from build123d import *

# Parameters (mm, degrees)
F1_DEPTH        = 34.5
F2_R            = 12.5
F3_DEPTH        = 4.1
F4_R            = 13
F5_DEPTH        = 4.1
F6_W            = 20.7
F6_H            = 29.8
F6_H_2          = 0.9
F7_DEPTH        = 31.9
F10_D           = 1.5
F10_DEPTH       = 5
F10_TIP         = 0.4506454643
F10_ON_F9_D     = 1.5
F10_ON_F9_DEPTH = 5
F10_ON_F9_TIP   = 0.4506454643
F12_DEPTH       = 25


with BuildPart() as f1:
    # F0 (on Front) → F1 (new body)
    with BuildSketch(Plane.XZ):
        Polygon((0, 36), (0, 0), (36, 0), (36, 5), (5, 36), align=None)
    extrude(amount=F1_DEPTH)

    # F2 (on face) → F3 (cut)
    with BuildSketch(Plane(origin=(0, 0, 0), x_dir=(0, -1, 0), z_dir=(-1, 0, 0))):
        with Locations((17.25, 18)):
            Circle(F2_R)
    extrude(amount=-F3_DEPTH, mode=Mode.SUBTRACT)

    # F4 (on face) → F5 (cut)
    with BuildSketch(Plane(origin=(0, 0, 0), x_dir=(1, 0, 0), z_dir=(0, 0, -1))):
        with Locations((18, 17.25)):
            Circle(F4_R)
    extrude(amount=-F5_DEPTH, mode=Mode.SUBTRACT)

    # F6 (on face) → F7 (cut)
    with BuildSketch(Plane.YZ.offset(36)):
        with Locations((-17.25, 19.9)):
            Rectangle(F6_W, F6_H)
        with Locations((-17.25, 4.55)):
            Rectangle(F6_W, F6_H_2)
    extrude(amount=-F7_DEPTH, mode=Mode.SUBTRACT)

    # F10
    with Locations(Plane.XY.offset(36)):
        with Locations((2.75, -31.75), (2.75, -2.75)):
            Hole(F10_D / 2, depth=F10_DEPTH)
            with Locations((0, 0, -(F10_DEPTH + F10_TIP / 2))):  # 118° drill point
                Cone(0, F10_D / 2, F10_TIP, mode=Mode.SUBTRACT)

    # F10 on F9
    with Locations(Plane.YZ.offset(36)):
        with Locations((-31.75, 2.75), (-2.75, 2.75)):
            Hole(F10_ON_F9_D / 2, depth=F10_ON_F9_DEPTH)
            with Locations((0, 0, -(F10_ON_F9_DEPTH + F10_ON_F9_TIP / 2))):  # 118° drill point
                Cone(0, F10_ON_F9_D / 2, F10_ON_F9_TIP, mode=Mode.SUBTRACT)

    # F11 (on face) → F12 (cut)
    with BuildSketch(Plane(origin=(0, 0, 0), x_dir=(0, -1, 0), z_dir=(-1, 0, 0))):
        with BuildLine():
            ThreePointArc((18, 5.5225202865), (17.5002003207, 5.5025042589), (17, 5.5025002501))
            Line((17, 5.5025002501), (17, 0))
            Line((17, 0), (18, 0))
            Line((18, 0), (18, 5.5225202865))
        make_face()
    extrude(amount=-F12_DEPTH, mode=Mode.SUBTRACT)


solid = f1.part
Design review of the part built by this model. Coordinates are the model's own, in mm. A direction names the side the tool comes from. Coordinates: 2 decimals unless noted, no trailing zeros. Order: outer loops, then holes, each group sorted by start corner. A loop starts at its lowest first (then second) coordinate and runs counter-clockwise, first axis right, second up. Notation, with made-up numbers: (46.25, 66.25) -> (52.25, 66.25) arc R31 ccw to (52.25, 93.25) -> close; hole circle Ø9 at (37, 2). An arc over 180 degrees is marked (long way). Use one line per item in the form item = value. Start each with the question number.
(1) Add section A-A on x = 18. State the section outline as (y, z) points.
(2) Add section C-C on y = -21.5. State the section outline as (x, z) points.
(3) Insertion check: pin 1 (8 mm diameter, centred on x = 32.5, y = -19.5, fed in from +Z); pin 2 (0.6 mm diameter, centred on y = -6, z = 15.5, fed in from -X); pin 3 (6 mm diameter, centred on x = 20, y = -7, fed in from +Z); pin 4 (3 mm diameter, centred on x = 31.5, z = 12, fed in from +Y). Each pin has a flat end and moves straight along its axis. Give the tip position at first contact, or say it passes through.
(4) For faces 5 (the flat face through (17, -27.6, 16)), 6 (the flat face through (2, -18, 3)), 7 (the flat face through (18, -29, 4.1)), 8 (the flat face through (4.1, -6, 18)), list the 3-axis set-ups (+Z, -Z, +X, -X, +Y, -Y) from which the entire face can be reached by the end or side of a thin tool; tool diameter is ignored.
(5) The part is to be moulded in two halves that separate along Z. For faces 1 (the flat face through (32, -17, 4.1)), 2 (the flat face through (18, -6, 4.1)), 3 (the cylindrical face through (33.465, -32.465, 2.975)), 4 (the flat face through (0, -13, 30)), say which applies: +Z half, -Z half, draft (parallel to the pull), parting line (faces both ways), or undercut.
(6) Add section B-B on z = 18. State the section outline as (x, y) points.
(7) Add section D-D on y = -14.5. State the section outline as (x, z) points, plus the area to 3 significant figures.
(8) For probe 1 along Y at (x, z) = (2.75, 34.05); probe 2 along Y at (x, z) = (16, 12); probe 3 along X at (y, z) = (-0.5, 16), list the stretches that pass through material, from the lowest coordinate up.
Answer block:
q1.outline = (-34.5, 0) -> (-30.25, 0) -> (-30.25, 4.1) -> (-27.6, 4.1) -> (-27.6, 23) -> (-34.5, 23) -> close; (-6.9, 4.1) -> (-4.25, 4.1) -> (-4.25, 0) -> (0, 0) -> (0, 23) -> (-6.9, 23) -> close
q2.outline = (0, 0) -> (5.71, 0) -> (5.71, 4.1) -> (4.1, 4.1) -> (4.1, 6.24) -> (0, 6.24) -> close; (0, 29.76) -> (4.1, 29.76) -> (4.1, 34.8) -> (6.2, 34.8) -> (5, 36) -> (0, 36) -> close; (30.29, 0) -> (36, 0) -> (36, 4.1) -> (30.29, 4.1) -> close
q3.pin_1 = 4.1
q3.pin_2 = 4.1
q3.pin_3 = 24
q3.pin_4 = through
q4.face_5 = +X
q4.face_6 = -Z, -X
q4.face_7 = -Z
q4.face_8 = -X
q5.face_1 = +Z half
q5.face_2 = -Z half
q5.face_3 = undercut
q5.face_4 = draft
q6.outline = (0, -34.5) -> (23, -34.5) -> (23, -27.6) -> (4.1, -27.6) -> (4.1, -29.75) -> (0, -29.75) -> close; (0, -4.75) -> (4.1, -4.75) -> (4.1, -6.9) -> (23, -6.9) -> (23, 0) -> (0, 0) -> close
q7.outline = (0, 0) -> (5.29, 0) -> (5.29, 4.1) -> (4.1, 4.1) -> (4.1, 5.81) -> (0, 5.81) -> close; (0, 30.19) -> (4.1, 30.19) -> (4.1, 34.8) -> (6.2, 34.8) -> (5, 36) -> (0, 36) -> close; (30.71, 0) -> (36, 0) -> (36, 4.1) -> (30.71, 4.1) -> close
q7.area = 76.0 mm²
q8.probe_1 = -34.5 to -32.5, -31 to -3.5, -2 to 0
q8.probe_2 = -34.5 to -27.6, -6.9 to 0
q8.probe_3 = 0 to 25
